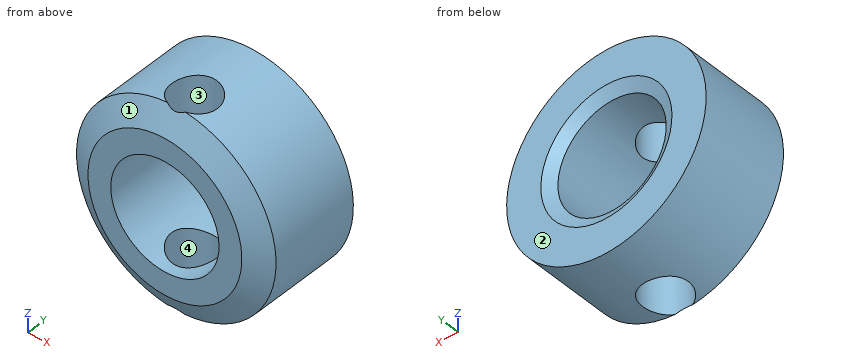
from build123d import *

# Parameters (mm, degrees)
SKETCH1_R               = 4.375
SKETCH1_R_2             = 2.375
BOSS_EXTRUDE1_DEPTH     = 4.5
CHAMFER1_SIZE           = 0.5
CHAMFER1_SIZE2          = 0.288675135
CHAMFER2_SIZE           = 1
CHAMFER2_SIZE2          = 0.577350269
CUT_EXTRUDE1_DEPTH      = 8.650571874
CUT_EXTRUDE1_DEPTH_BACK = 8.650571874
SKETCH2_R               = 1


with BuildPart() as part:
    # Sketch1 → Boss-Extrude1 (new body)
    with BuildSketch(Plane(origin=(0, 0, 0), x_dir=(1, 0, 0), z_dir=(0, 1, 0))):
        with Locations(Location((0, 0, 0), (0, 0, 270))):
            Circle(SKETCH1_R)
        with Locations(Location((0, 0, 0), (0, 0, 270))):
            Circle(SKETCH1_R_2, mode=Mode.SUBTRACT)
    extrude(amount=BOSS_EXTRUDE1_DEPTH)

    # Chamfer1
    chamfer1_edges = [part.edges().sort_by_distance(p)[0] for p in [
        (0, 4.5, -2.375),
    ]]
    chamfer1_side = [part.faces().sort_by_distance(p)[0] for p in [
        (0, 4.5, -4.251256313),
    ]]
    chamfer(chamfer1_edges, length=CHAMFER1_SIZE, length2=CHAMFER1_SIZE2, reference=chamfer1_side[0])

    # Chamfer2
    chamfer2_edges = [part.edges().sort_by_distance(p)[0] for p in [
        (0, 0, -4.375),
    ]]
    chamfer2_side = [part.faces().sort_by_distance(p)[0] for p in [
        (0, 0, -4.251256313),
    ]]
    chamfer(chamfer2_edges, length=CHAMFER2_SIZE, length2=CHAMFER2_SIZE2, reference=chamfer2_side[0])

    # Sketch2 → Cut-Extrude1 (cut, two sides: drawn at the far end of the back side and taken through both)
    with BuildSketch(Plane.XY.offset(-CUT_EXTRUDE1_DEPTH_BACK)):
        with Locations(Location((0, 1.5, 0), (0, 0, 292.683630924))):
            Circle(SKETCH2_R)
    extrude(amount=CUT_EXTRUDE1_DEPTH + CUT_EXTRUDE1_DEPTH_BACK, mode=Mode.SUBTRACT)


solid = part.part
Work out the finished part from the listing and answer in its coordinate system (mm). Face numbers are marked on the shaded views. Round coordinates to 2 decimals unless told otherwise and drop trailing zeros. Write each loop counter-clockwise with the first axis right and the second up, starting at its lowest first coordinate (ties: lowest second). Pieces come first, ordered by that corner, then holes. Notation, with made-up numbers: (46, 3.25) -> (71, 3.25) arc R14 cw to (71, 17.25) -> close; hole circle Ø1 at (65.5, -6.75). An arc over 180 degrees is marked (long way). Answer as CSV lines item,"result". Start each with the question number.
(1) The mould has two halves that part along Y. Classify the marked faces 1, 2, 3 and 4: +Y half, -Y half, draft (parallel to the pull), parting line (faces both ways), or undercut.
(2) Find the intervals of material crossed by probe 1 along Y at (x, z) = (0, 3.25); probe 2 along X at (y, z) = (2.05, 0) (3 decimals); probe 3 along X at (y, z) = (1.5, -3.3), in increasing order.
(3) The part is cut by section A-A, the plane z = 0. Give the vertices of the cut face in (x, y) (3 decimals).
(4) The part is cut by section B-B, the plane x = 0. Give the vertices of the cut face in (y, z) (3 decimals), then the cut area to 3 significant figures.
(5) Each of these flat-tipped pins is pushed along its axis until it touches: pin 1 (1.6 mm diameter, centred on x = 0, y = 1.5, fed in from -Z); pin 2 (2 mm diameter, centred on x = -1.5, y = 3.5, fed in from -Z); pin 3 (2 mm diameter, centred on y = 2.5, z = 2, fed in from -X). Where does it stop, or does it pass through?
(6) The part is cut by section D-D, the plane y = 3.4. Give the vertices of the cut face in (x, z) (3 decimals).
(7) The part is cut by section C-C, the plane y = 1.1. Give the vertices of the cut face in (x, z) (3 decimals).
Output values:
1,face 1,"-Y half"
1,face 2,"+Y half"
1,face 3,"undercut"
1,face 4,"undercut"
2,probe 1,"y = 0 to 0.5, 2.5 to 4.5"
2,probe 2,"x = -4.375 to -2.375, 2.375 to 4.375"
2,probe 3,"x = -2.87 to -1, 1 to 2.87"
3,outline,"(-4.375, 0.577) -> (-3.375, 0) -> (-2.375, 0) -> (-2.375, 4.211) -> (-2.875, 4.5) -> (-4.375, 4.5) -> close; (2.375, 0) -> (3.375, 0) -> (4.375, 0.577) -> (4.375, 4.5) -> (2.875, 4.5) -> (2.375, 4.211) -> close"
4,outline,"(0, -3.375) -> (0.5, -4.241) -> (0.5, -2.375) -> (0, -2.375) -> close; (0, 2.375) -> (0.5, 2.375) -> (0.5, 4.241) -> (0, 3.375) -> close; (2.5, -4.375) -> (4.5, -4.375) -> (4.5, -2.875) -> (4.211, -2.375) -> (2.5, -2.375) -> close; (2.5, 2.375) -> (4.211, 2.375) -> (4.5, 2.875) -> (4.5, 4.375) -> (2.5, 4.375) -> close"
4,area,"9.29 mm²"
5,pin 1,"passes through"
5,pin 2,"stops at z = -4.35"
5,pin 3,"stops at x = -4.26"
6,outline,"circle Ø8.75 at (0, 0); hole circle Ø4.75 at (0, 0)"
7,outline,"(-0.917, -4.278) -> (-0.917, -2.191) arc R2.375 cw to (-0.917, 2.191) -> (-0.917, 4.278) arc R4.375 ccw to start; (0.917, -4.278) arc R4.375 ccw to (0.917, 4.278) -> (0.917, 2.191) arc R2.375 cw to (0.917, -2.191) -> close"
